Job drawing, mm, ordinate dimensions from the low corner. One solid piece. Coordinates: 2 decimals unless noted, no trailing zeros. Write each loop counter-clockwise with the first axis right and the second up, starting at its lowest first coordinate (ties: lowest second). Pieces come first, ordered by that corner, then holes. Notation, with made-up numbers: (-20, 71) - (14, 71) arc R32 ccw to (14, 105) - close; hole circle Ø5 at (20.25, -3). An arc over 180 degrees is marked (long way). Use a Markdown table: item, result.
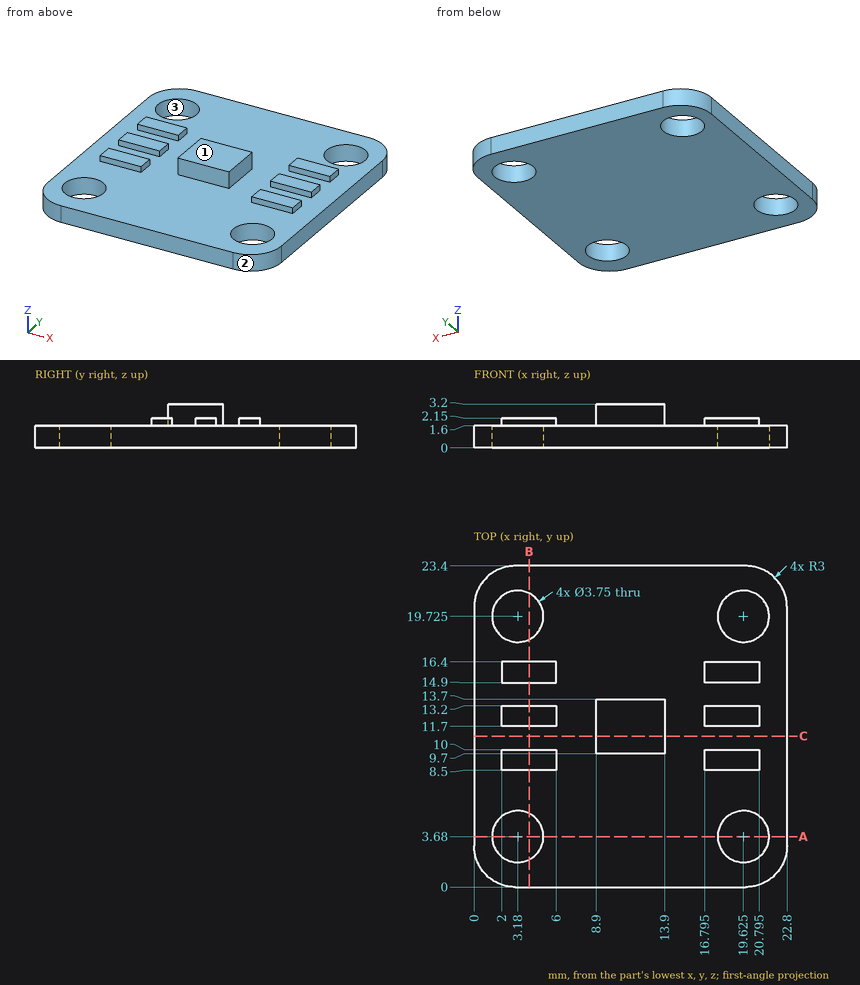
Item 1: Drill centre lines: probe 1 along Y at (x, z) = (2.75, 1.7); probe 2 along Y at (x, z) = (19.75, 0.8); probe 3 along X at (y, z) = (3.5, 1.45). Where is each one in solid material? Low to high.
From the geometry:
| item | result |
|---|---|
| probe 1 | 8.5 to 10, 11.7 to 13.2, 14.9 to 16.4 |
| probe 2 | 0 to 1.81, 5.55 to 17.85, 21.6 to 23.4 |
| probe 3 | 0 to 1.31, 5.05 to 17.76, 21.49 to 22.8 |
Item 2: Two-plate mould, pull along X, no slides. Class the marked faces 1, 2 and 3: pulls with the +X half, pulls with the -X half, needs draft (parallel to the pull), parting line crosses it, or undercut.
From the geometry:
| item | result |
|---|---|
| face 1 | needs draft |
| face 2 | pulls with the +X half |
| face 3 | undercut |
Item 3: Band-saw the part on C-C, the plane y = 11. Give the cut face in (x, z).
From the geometry:
| item | result |
|---|---|
| outline | (0, 0) - (22.8, 0) - (22.8, 1.6) - (13.9, 1.6) - (13.9, 3.2) - (8.9, 3.2) - (8.9, 1.6) - (0, 1.6) - close |
Item 4: Drop flat-ended pins along their axis: P1, Ø1.2, axis at x = 18.5, y = 9, coming from the +Z side; P2, Ø0.5, axis at y = 11.5, z = 2.5, coming from the +X side; P3, Ø0.6, axis at y = 9.5, z = 2, coming from the +X side (1 decimal). Give the stop position or say it passes through.
From the geometry:
| item | result |
|---|---|
| P1 | z = 2.15 |
| P2 | x = 13.9 |
| P3 | x = 20.8 |
Item 5: Band-saw the part on A-A, the plane y = 3.68. Count the separate pieces of the cut face and the enclosed holes in it, then the cut area to 3 significant figures.
From the geometry:
| item | result |
|---|---|
| separate pieces | 3 |
| enclosed holes | 0 |
| area | 24.5 mm^2 |
Item 6: Band-saw the part on B-B, the plane x = 4. Give the cut face in (y, z).
From the geometry:
| item | result |
|---|---|
| outline | (0, 0) - (1.99, 0) - (1.99, 1.6) - (0, 1.6) - close; (5.37, 0) - (18.04, 0) - (18.04, 1.6) - (16.4, 1.6) - (16.4, 2.15) - (14.9, 2.15) - (14.9, 1.6) - (13.2, 1.6) - (13.2, 2.15) - (11.7, 2.15) - (11.7, 1.6) - (10, 1.6) - (10, 2.15) - (8.5, 2.15) - (8.5, 1.6) - (5.37, 1.6) - close; (21.41, 0) - (23.4, 0) - (23.4, 1.6) - (21.41, 1.6) - close |
